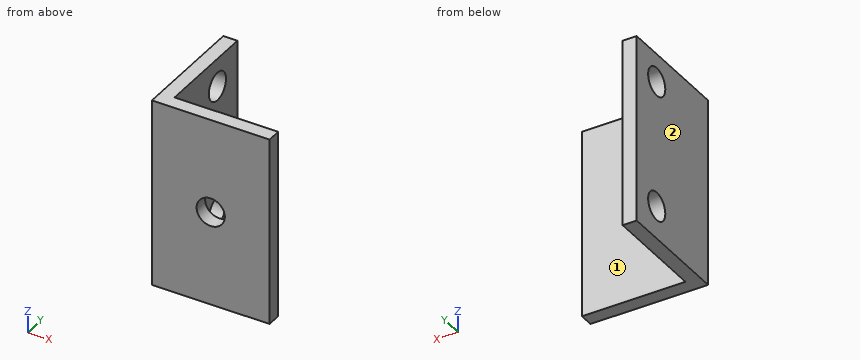
```python
from build123d import *

# Parameters (mm, degrees)
SALIENTE_EXTRUIR1_DEPTH = 20
CROQUIS2_R              = 1.5
CORTAR_EXTRUIR1_DEPTH   = 1.5
CROQUIS3_R              = 1.5
CORTAR_EXTRUIR2_DEPTH   = 1.5


with BuildPart() as part:
    # Croquis1 → Saliente-Extruir1 (new body)
    with BuildSketch(Plane.XY):
        Polygon((0, 0), (12.5, 0), (12.5, 1.5), (1.5, 1.5), (1.5, 12.5), (0, 12.5), align=None)
    extrude(amount=SALIENTE_EXTRUIR1_DEPTH)

    # Croquis2 → Cortar-Extruir1 (cut)
    with BuildSketch(Plane.ZY):
        with Locations(Location((17, 9, 0), (0, 0, 270))):
            Circle(CROQUIS2_R)
        with Locations(Location((3.5, 9, 0), (0, 0, 270))):
            Circle(CROQUIS2_R)
    extrude(amount=-CORTAR_EXTRUIR1_DEPTH, mode=Mode.SUBTRACT)

    # Croquis3 → Cortar-Extruir2 (cut)
    with BuildSketch(Plane.XZ):
        with Locations(Location((6.25, 10, 0), (0, 0, 270))):
            Circle(CROQUIS3_R)
    extrude(amount=-CORTAR_EXTRUIR2_DEPTH, mode=Mode.SUBTRACT)


solid = part.part
```
Here's how the part is built. I have some questions about the finished solid (model axes, mm). Face numbers are marked on the shaded views. A direction names the side the tool comes from. Coordinates: 2 decimals unless noted, no trailing zeros. Order: outer loops, then holes, each group sorted by start corner. A loop starts at its lowest first (then second) coordinate and runs counter-clockwise, first axis right, second up.
Item 1: I'm going to push flat-ended pins straight in: pin 1 Ø1.5 at (y, z) = (6.5, 9) entering from +X; pin 2 Ø2 at (x, z) = (11, 15.5) entering from +Y. Where does each tip first touch, or does it pass through?
Response values:
pin 1: stops at x = 1.5
pin 2: stops at y = 1.5
Item 2: If we section it at B-B, the plane z = 17: List the corners of the cut face in (x, y) for me, then the cut area to 4 significant figures.
Response values:
outline: (0, 0) - (12.5, 0) - (12.5, 1.5) - (1.5, 1.5) - (1.5, 7.5) - (0, 7.5) - close; (0, 10.5) - (1.5, 10.5) - (1.5, 12.5) - (0, 12.5) - close
area: 30.75 mm2
Item 3: I need wall thicknesses on probe 1 along Z at (x, y) = (0.45, 9); probe 2 along X at (y, z) = (0.7, 10); probe 3 along X at (y, z) = (3.25, 9.5). Which ranges of each line are inside material? Lowest first, please.
Response values:
probe 1: z = 0 to 2, 5 to 15.5, 18.5 to 20
probe 2: x = 0 to 4.75, 7.75 to 12.5
probe 3: x = 0 to 1.5
Item 4: If we section it at D-D, the plane z = 9.25: List the corners of the cut face in (x, y) for me.
Response values:
outline: (0, 0) - (4.95, 0) - (4.95, 1.5) - (1.5, 1.5) - (1.5, 12.5) - (0, 12.5) - close; (7.55, 0) - (12.5, 0) - (12.5, 1.5) - (7.55, 1.5) - close
Item 5: If we section it at C-C, the plane x = 6.75: List the corners of the cut face in (y, z) for me, then the cut area to 3 significant figures.
Response values:
outline: (0, 0) - (1.5, 0) - (1.5, 8.59) - (0, 8.59) - close; (0, 11.41) - (1.5, 11.41) - (1.5, 20) - (0, 20) - close
area: 25.8 mm2
Item 6: Which directions (+Z, -Z, +X, -X, +Y, -Y) give clear straight access to the entire face, cutting with the end or side of a thin tool? Please do the marked faces 1 and 2.
Response values:
face 1: +Z, -Z, +X, +Y
face 2: +Z, -Z, -X, +Y, -Y
Item 7: If we section it at A-A, the plane y = 9: List the corners of the cut face in (x, z) for me, then the cut area to 3 significant figures.
Response values:
outline: (0, 0) - (1.5, 0) - (1.5, 2) - (0, 2) - close; (0, 5) - (1.5, 5) - (1.5, 15.5) - (0, 15.5) - close; (0, 18.5) - (1.5, 18.5) - (1.5, 20) - (0, 20) - close
area: 21.0 mm2
